Study the drawing (mm; zero at the part's minimum x, y, z) and answer. Coordinates: 2 decimals unless noted, no trailing zeros. Order: outer loops, then holes, each group sorted by start corner. A loop starts at its lowest first (then second) coordinate and runs counter-clockwise, first axis right, second up. Notation, with made-up numbers: (-33, 61.5) - (-27, 61.5) arc R24 cw to (-27, 80.5) - close; hole circle Ø6 at (78.25, -1). An arc over 180 degrees is marked (long way). Write item = value, one per line.
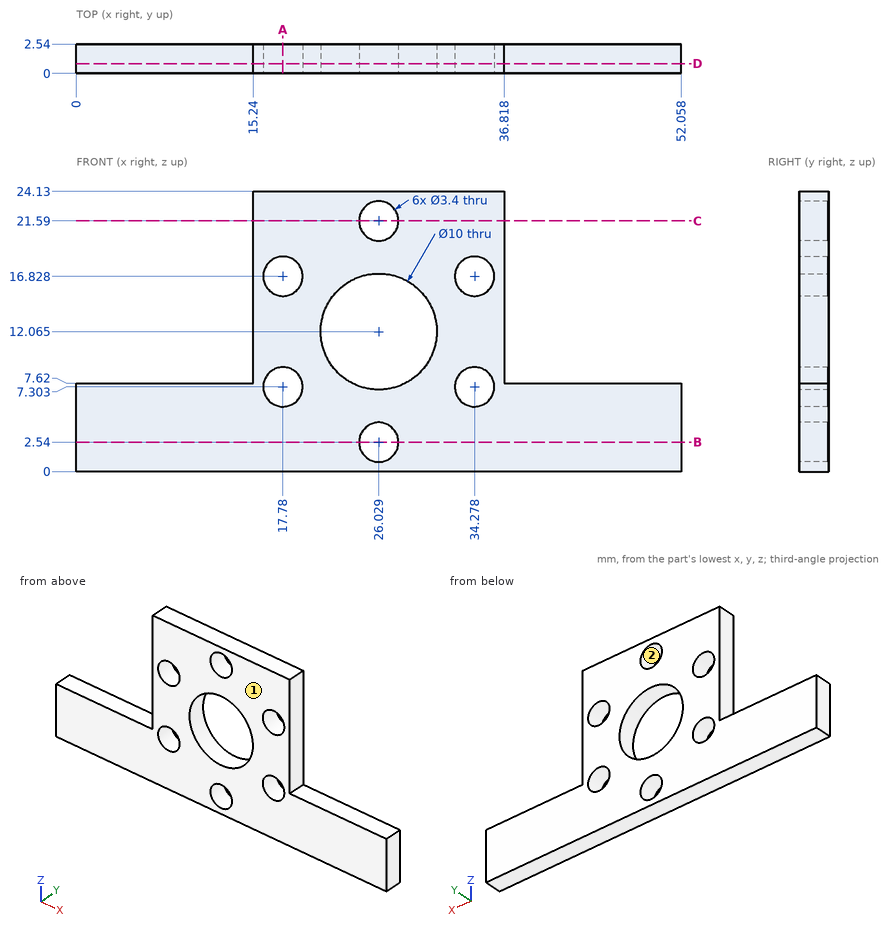
1) Determine the mould class of the marked faces 1 and 2 for opening direction Z: pulls with the +Z half, pulls with the -Z half, needs draft (parallel to the pull), parting line crosses it, or undercut.
Returned:
face_1 = needs draft
face_2 = undercut
2) The part is cut by section C-C (z = 21.59). Determine the outline of the cut face in (x, y).
Returned:
outline = (15.24, 0) - (24.33, 0) - (24.33, 2.54) - (15.24, 2.54) - close; (27.73, 0) - (36.82, 0) - (36.82, 2.54) - (27.73, 2.54) - close
3) Flat-ended cylindrical pins translate along their axes: pin 1 Ø8 at (x, z) = (26.03, 12.06) entering from +Y; pin 2 Ø1.3 at (x, y) = (44, 2) entering from +Z; pin 3 Ø1.5 at (y, z) = (0.5, 13) entering from +X. Find the tip coordinate at first contact, or state that the pin passes through.
Returned:
pin_1 = through
pin_2 = 7.62
pin_3 = 36.82
4) The part is cut by section B-B (z = 2.54). Determine the outline of the cut face in (x, y).
Returned:
outline = (0, 0) - (24.33, 0) - (24.33, 2.54) - (0, 2.54) - close; (27.73, 0) - (52.06, 0) - (52.06, 2.54) - (27.73, 2.54) - close
5) Straight lines are drawn through the part: line 1 along Z through (x, y) = (17.78, 0.65); line 2 along X through (y, z) = (1, 6.25) (1 decimal); line 3 along X through (y, z) = (1.25, 5.75) (1 decimal). For each, find the intervals that lie inside material, in ascending order. Write a range as from..to.
Returned:
line_1 = 0..5.6, 9..15.13, 18.53..24.13
line_2 = 0..16.4, 19.1..32.9, 35.6..52.1
line_3 = 0..17.1, 18.5..33.6, 35..52.1
6) The part is cut by section A-A (x = 17.78). Determine the outline of the cut face in (y, z).
Returned:
outline = (0, 0) - (2.54, 0) - (2.54, 5.6) - (0, 5.6) - close; (0, 9) - (2.54, 9) - (2.54, 15.13) - (0, 15.13) - close; (0, 18.53) - (2.54, 18.53) - (2.54, 24.13) - (0, 24.13) - close
7) The part is cut by section D-D (y = 0.85). Determine the outline of the cut face in (x, z) (1 decimal).
Returned:
outline = (0, 0) - (52.1, 0) - (52.1, 7.6) - (36.8, 7.6) - (36.8, 24.1) - (15.2, 24.1) - (15.2, 7.6) - (0, 7.6) - close; hole circle Ø3.4 at (17.8, 7.3); hole circle Ø3.4 at (17.8, 16.8); hole circle Ø10 at (26, 12.1); hole circle Ø3.4 at (26, 2.5); hole circle Ø3.4 at (26, 21.6); hole circle Ø3.4 at (34.3, 7.3); hole circle Ø3.4 at (34.3, 16.8)
